Autodesk Fusion 360 part; units mm, degrees
sketch "スケッチ1" plane through (0, 0, 0) normal (0, 1, 0) x (1, 0, 0)
  line L0 (8, 10) -> (-8, 10)
  line L1 (-10, 8) -> (-10, -8)
  line L2 (-8, -10) -> (8, -10)
  line L3 (10, -8) -> (10, 8)
  line L4 (10, 10) -> (-10, -10) construction
  line L5 (-10, 10) -> (10, -10) construction
  circle A0 centre (0, 0) radius 2.6
  line L6 (-3.2, -10) -> (-3.2, -8.65)
  line L7 (-3.2, -8.65) -> (-4.6, -8.65)
  line L8 (-5.1, -8.15) -> (-5.1, -6.3678)
  line L9 (-4.9536, -6.0142) -> (-3.4251, -4.4858)
  line L10 (0, 0) -> (0, -10) construction
  line L11 (-2.0109, -3.9) -> (0, -3.9)
  arc A1 (-5.1, -8.15) -> (-4.6, -8.65) centre (-4.6, -8.15) ccw
  arc A2 (-4.9536, -6.0142) -> (-5.1, -6.3678) centre (-4.6, -6.3678) ccw
  arc A3 (-2.0109, -3.9) -> (-3.4251, -4.4858) centre (-2.0109, -5.9) ccw
  arc A4 (-10, -8) -> (-8, -10) centre (-8, -8) ccw
  arc A5 (10, 8) -> (8, 10) centre (8, 8) ccw
  arc A6 (8, -10) -> (10, -8) centre (8, -8) ccw
  arc A7 (-8, 10) -> (-10, 8) centre (-8, 8) ccw
  line L12 (3.2, -10) -> (3.2, -8.65)
  line L13 (3.2, -8.65) -> (4.6, -8.65)
  arc A8 (4.6, -8.65) -> (5.1, -8.15) centre (4.6, -8.15) ccw
  line L14 (5.1, -8.15) -> (5.1, -6.3678)
  arc A9 (5.1, -6.3678) -> (4.9536, -6.0142) centre (4.6, -6.3678) ccw
  line L15 (4.9536, -6.0142) -> (3.4251, -4.4858)
  arc A10 (3.4251, -4.4858) -> (2.0109, -3.9) centre (2.0109, -5.9) ccw
  line L16 (2.0109, -3.9) -> (0, -3.9)
  line L17 (10, -3.2) -> (8.65, -3.2)
  line L18 (8.65, -3.2) -> (8.65, -4.6)
  arc A11 (8.15, -5.1) -> (8.65, -4.6) centre (8.15, -4.6) ccw
  line L19 (8.15, -5.1) -> (6.3678, -5.1)
  arc A12 (6.0142, -4.9536) -> (6.3678, -5.1) centre (6.3678, -4.6) ccw
  line L20 (6.0142, -4.9536) -> (4.4858, -3.4251)
  arc A13 (3.9, -2.0109) -> (4.4858, -3.4251) centre (5.9, -2.0109) ccw
  line L21 (3.9, -2.0109) -> (3.9, 0)
  line L22 (3.9, 2.0109) -> (3.9, 0)
  arc A14 (4.4858, 3.4251) -> (3.9, 2.0109) centre (5.9, 2.0109) ccw
  line L23 (6.0142, 4.9536) -> (4.4858, 3.4251)
  arc A15 (6.3678, 5.1) -> (6.0142, 4.9536) centre (6.3678, 4.6) ccw
  line L24 (8.15, 5.1) -> (6.3678, 5.1)
  arc A16 (8.65, 4.6) -> (8.15, 5.1) centre (8.15, 4.6) ccw
  line L25 (8.65, 3.2) -> (8.65, 4.6)
  line L26 (10, 3.2) -> (8.65, 3.2)
  line L27 (3.2, 10) -> (3.2, 8.65)
  line L28 (3.2, 8.65) -> (4.6, 8.65)
  arc A17 (5.1, 8.15) -> (4.6, 8.65) centre (4.6, 8.15) ccw
  line L29 (5.1, 8.15) -> (5.1, 6.3678)
  arc A18 (4.9536, 6.0142) -> (5.1, 6.3678) centre (4.6, 6.3678) ccw
  line L30 (4.9536, 6.0142) -> (3.4251, 4.4858)
  arc A19 (2.0109, 3.9) -> (3.4251, 4.4858) centre (2.0109, 5.9) ccw
  line L31 (2.0109, 3.9) -> (0, 3.9)
  line L32 (-2.0109, 3.9) -> (0, 3.9)
  arc A20 (-3.4251, 4.4858) -> (-2.0109, 3.9) centre (-2.0109, 5.9) ccw
  line L33 (-4.9536, 6.0142) -> (-3.4251, 4.4858)
  arc A21 (-5.1, 6.3678) -> (-4.9536, 6.0142) centre (-4.6, 6.3678) ccw
  line L34 (-5.1, 8.15) -> (-5.1, 6.3678)
  arc A22 (-4.6, 8.65) -> (-5.1, 8.15) centre (-4.6, 8.15) ccw
  line L35 (-3.2, 8.65) -> (-4.6, 8.65)
  line L36 (-3.2, 10) -> (-3.2, 8.65)
  line L37 (-10, 3.2) -> (-8.65, 3.2)
  line L38 (-8.65, 3.2) -> (-8.65, 4.6)
  arc A23 (-8.15, 5.1) -> (-8.65, 4.6) centre (-8.15, 4.6) ccw
  line L39 (-8.15, 5.1) -> (-6.3678, 5.1)
  arc A24 (-6.0142, 4.9536) -> (-6.3678, 5.1) centre (-6.3678, 4.6) ccw
  line L40 (-6.0142, 4.9536) -> (-4.4858, 3.4251)
  arc A25 (-3.9, 2.0109) -> (-4.4858, 3.4251) centre (-5.9, 2.0109) ccw
  line L41 (-3.9, 2.0109) -> (-3.9, 0)
  line L42 (-3.9, -2.0109) -> (-3.9, 0)
  arc A26 (-4.4858, -3.4251) -> (-3.9, -2.0109) centre (-5.9, -2.0109) ccw
  line L43 (-6.0142, -4.9536) -> (-4.4858, -3.4251)
  arc A27 (-6.3678, -5.1) -> (-6.0142, -4.9536) centre (-6.3678, -4.6) ccw
  line L44 (-8.15, -5.1) -> (-6.3678, -5.1)
  arc A28 (-8.65, -4.6) -> (-8.15, -5.1) centre (-8.15, -4.6) ccw
  line L45 (-8.65, -3.2) -> (-8.65, -4.6)
  line L46 (-10, -3.2) -> (-8.65, -3.2)
  dimension "d1" = 20
  dimension "d2" = 20
  dimension "d3" = 5.2
  dimension "d4" = 1.35
  dimension "d5" = 3.2
  dimension "d6" = 5.1
  dimension "d7" = 6.1
  dimension "d8" = 0.75
  dimension "d9" = 0.5
  dimension "d10" = 2
  dimension "d11" = 2
  dimension "d12" = 2
  dimension "d13" = 2
  dimension "d14" = 2
  dimension "d16" = 360
extrude "押し出し1" add sketch "スケッチ1" along normal mid plane 140 contours L0 L1 L2 L3 L6 L7 L8 L9 L11 A1 A2 A3 A4 A5 A6 A7 L12 L13 A8 L14 A9 L15 A10 L16 L17 L18 A11 L19 A12 L20 A13 L21 L22 A14 L23 A15 L24 A16 L25 L26 L27 L28 A17 L29 A18 L30 A19 L31 L32 A20 L33 A21 L34 A22 L35 L36 L37 L38 A23 L39 A24 L40 A25 L41 L42 A26 L43 A27 L44 A28 L45 L46
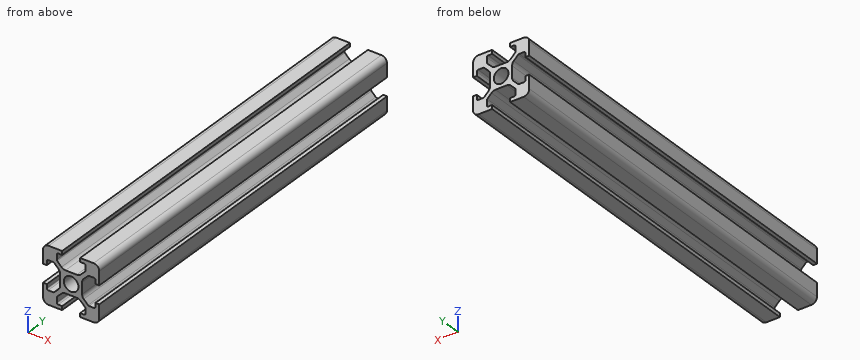
Verification items for the finished model (mm, model axes). Round coordinates to 2 decimals unless told otherwise and drop trailing zeros. Loops run counter-clockwise (first coordinate to the right, second up) from the corner with the lowest first, then second, coordinate; pieces in that order, holes last. Notation, with made-up numbers: (22, -8.75) - (52, -8.75) arc R17 cw to (52, 22.25) - close; hole circle Ø9 at (-1, 58.5). An arc over 180 degrees is marked (long way). Use one line per item in the form item = value.
1. Gauge pin test, flat ends, axial feed: pin 1 Ø1.5 at (x, y) = (-9.5, -22.5) entering from +Z; pin 2 Ø1.5 at (y, z) = (-34, 9) entering from -X; pin 3 Ø4 at (x, y) = (-3, -48.5) entering from +Z; pin 4 Ø1.1 at (y, z) = (-32.5, -9.5) entering from +X. Record the tip position at first contact, or that the pin passes through.
A:
pin_1 = 9.85
pin_2 = -9.98
pin_3 = 10
pin_4 = 9.76
2. Scan lines: probe 1 along Z at (x, y) = (-6.5, 6.5); probe 2 along X at (y, z) = (17, -4.25); probe 3 along Z at (x, y) = (0, -5). Record each from-to range of solid material in increasing order.
A:
probe_1 = -10 to -5.1, 5.1 to 10
probe_2 = -10 to -8.65, -5.31 to -3.14, 3.14 to 5.31, 8.65 to 10
probe_3 = -3.9 to -2.6, 2.6 to 3.9
3. Section check A-A on z = 0. Record the cut outline in (x, y), and give its area (3 significant figures).
A:
outline = (-3.9, -70) - (-2.6, -70) - (-2.6, 70) - (-3.9, 70) - close; (2.6, -70) - (3.9, -70) - (3.9, 70) - (2.6, 70) - close
area = 364 mm²
4. Section check B-B on x = 0. Record the cut outline in (y, z).
A:
outline = (-70, -3.9) - (70, -3.9) - (70, -2.6) - (-70, -2.6) - close; (-70, 2.6) - (70, 2.6) - (70, 3.9) - (-70, 3.9) - close
